Verification items for this drawing (mm, ordinates from the low corner). Coordinates: 2 decimals unless noted, no trailing zeros. Write each loop counter-clockwise with the first axis right and the second up, starting at its lowest first coordinate (ties: lowest second). Pieces come first, ordered by that corner, then holes. Notation, with made-up numbers: (52, 11.5) -> (64, 11.5) arc R29 ccw to (64, 48.5) -> close; hole circle Ø2 at (88.25, 54.5). An arc over 180 degrees is marked (long way). Put each result on its own line as item: value. Start each with the question number.
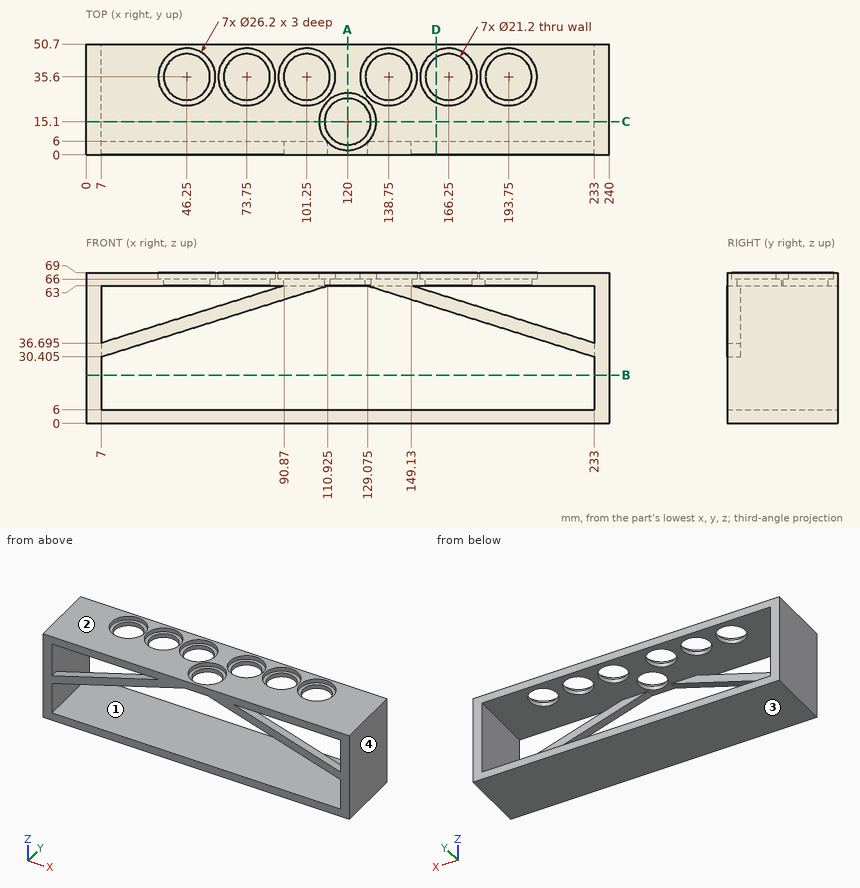
Item 1: Section check C-C, the plane y = 15.1. Enter the section's corners in (x, z).
Item 2: Scan lines: line 1 along Z through (x, y) = (193, 10); line 2 along X through (y, z) = (39, 38); line 3 along X through (y, z) = (15, 64). Record each from-to range of solid material in increasing order. Write a range as [from, to].
Item 3: Section check B-B, the plane z = 22. Enter the section's corners in (x, y).
Item 4: Go/stop test with flat-tipped pins: P1, Ø1.5, axis at x = 154, y = 35, coming from the -Z side; P2, Ø8, axis at x = 199.5, y = 38, coming from the +Z side; P3, Ø8, axis at x = 91, z = 11, coming from the +Y side; P4, Ø6, axis at x = 141, y = 27.5, coming from the +Z side. Record where each tip stops, or that it passes through.
Item 5: Mould release check, pull along Z, two halves, no side actions. Record for the marked faces 1, 2, 3 and 4: released by +Z, released by -Z, zero draft, split by the parting line, or undercut.
Item 6: Section check A-A, the plane x = 120. Enter the section's corners in (y, z), and give its area (3 significant figures).
Item 7: Section check D-D, the plane x = 160.5. Enter the section's corners in (y, z) (1 decimal), and give its area (3 significant figures).
From the geometry:
1. outline: (0, 0) -> (240, 0) -> (240, 69) -> (133.1, 69) -> (133.1, 66) -> (130.6, 66) -> (130.6, 63) -> (233, 63) -> (233, 6) -> (7, 6) -> (7, 63) -> (109.4, 63) -> (109.4, 66) -> (106.9, 66) -> (106.9, 69) -> (0, 69) -> close
2. line 1: [0, 6], [63, 69]
2. line 2: [0, 7], [233, 240]
2. line 3: [0, 109.4], [130.6, 240]
3. outline: (0, 0) -> (7, 0) -> (7, 50.7) -> (0, 50.7) -> close; (233, 0) -> (240, 0) -> (240, 50.7) -> (233, 50.7) -> close
4. P1: z = 0
4. P2: z = 6
4. P3: through
4. P4: z = 66
5. face 1: undercut
5. face 2: released by +Z
5. face 3: released by -Z
5. face 4: zero draft
6. outline: (0, 0) -> (50.7, 0) -> (50.7, 6) -> (0, 6) -> close; (0, 63) -> (4.5, 63) -> (4.5, 66) -> (2, 66) -> (2, 69) -> (0, 69) -> close; (25.7, 63) -> (50.7, 63) -> (50.7, 69) -> (28.2, 69) -> (28.2, 66) -> (25.7, 66) -> close
6. area: 466 mm²
7. outline: (0, 0) -> (50.7, 0) -> (50.7, 6) -> (0, 6) -> close; (0, 53.1) -> (6, 53.1) -> (6, 59.4) -> (0, 59.4) -> close; (0, 63) -> (26.7, 63) -> (26.7, 66) -> (23.8, 66) -> (23.8, 69) -> (0, 69) -> close; (44.5, 63) -> (50.7, 63) -> (50.7, 69) -> (47.4, 69) -> (47.4, 66) -> (44.5, 66) -> close
7. area: 522 mm²
